For this review, take the finished solid that the model builds, in its own axes (mm). Face numbers are marked on the shaded views. A direction names the side the tool comes from. Coordinates: 2 decimals unless noted, no trailing zeros. Write each loop counter-clockwise with the first axis right and the second up, starting at its lowest first coordinate (ties: lowest second). Pieces come first, ordered by that corner, then holes. Notation, with made-up numbers: (-36.5, 87) -> (-20.5, 87) arc R5 cw to (-20.5, 96) -> close; hole circle Ø7 at (-32, 1.25). An arc over 180 degrees is marked (long way). One line per item, written item: value. Start each with the question number.
1) Machinability: for the marked faces 1 and 2, which of the approach directions +Z, -Z, +X, -X, +Y, -Y give a long, thin tool a straight path to every point of the face, cutting with its end or side? Answer none if there is none.
2) Add section A-A (x = 58.5). State the section outline as (y, z) points, and give its area (3 significant figures).
3) For pin 1 Ø12 at (y, z) = (75, 142.5) entering from -X; pin 2 Ø12 at (x, y) = (269, 199) entering from +Z, all flat-tipped, find the tip position at first contact; note any pin that passes through.
4) Add section B-B (y = 203.5). State the section outline as (x, z) points.
5) For probe 1 along Z at (x, y) = (232, 227), list the stretches that pass through material, from the lowest coordinate up. Write a range as from..to.
6) Add section C-C (x = 122). State the section outline as (y, z) points, and give its area (3 significant figures).
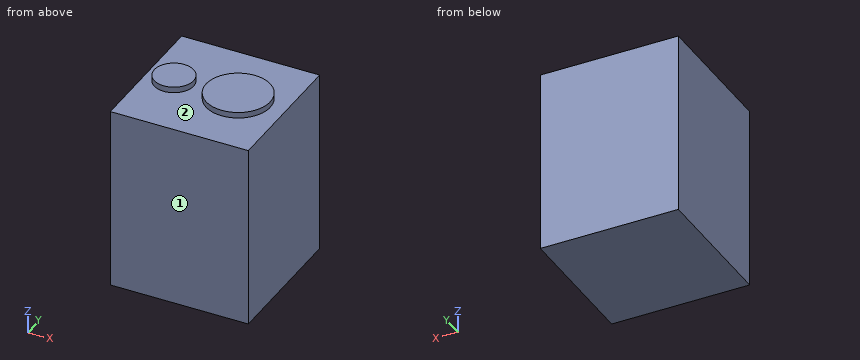
from build123d import *

# Parameters (mm, degrees)
SKETCH1_W           = 300
SKETCH1_H           = 300
BOSS_EXTRUDE1_DEPTH = 400
SKETCH2_R           = 42.704595991
SKETCH2_R_2         = 69.587993354
BOSS_EXTRUDE2_DEPTH = 12.7


with BuildPart() as part:
    # Sketch1 → Boss-Extrude1 (new body)
    with BuildSketch(Plane.XY):
        with Locations((150, 150)):
            Rectangle(SKETCH1_W, SKETCH1_H)
    extrude(amount=BOSS_EXTRUDE1_DEPTH)

    # Sketch2 → Boss-Extrude2 (add)
    with BuildSketch(Plane.XY.offset(400)):
        with Locations(Location((59.050998503, 153.288809659, 0), (0, 0, 180))):
            Circle(SKETCH2_R)
        with Locations(Location((197.894381645, 154.860769066, 0), (0, 0, 180))):
            Circle(SKETCH2_R_2)
    extrude(amount=BOSS_EXTRUDE2_DEPTH)


solid = part.part
Numbers:
1. face 1: +Z, -Z, +X, -X, -Y
1. face 2: +Z
2. outline: (0, 0) -> (300, 0) -> (300, 400) -> (195.99, 400) -> (195.99, 412.7) -> (110.59, 412.7) -> (110.59, 400) -> (0, 400) -> close
2. area: 121,000 mm²
3. pin 1: x = 0
3. pin 2: z = 400
4. outline: (0, 0) -> (300, 0) -> (300, 400) -> (247.66, 400) -> (247.66, 412.7) -> (148.13, 412.7) -> (148.13, 400) -> (0, 400) -> close
5. probe 1: 0..400
6. outline: (0, 0) -> (300, 0) -> (300, 400) -> (0, 400) -> close
6. area: 120,000 mm²
